Geometry check sheet. Reference: the model listing, model coordinates, mm. A direction names the side the tool comes from. Give positions to 0.01 mm unless a question says otherwise; leave off trailing zeros. Order: outer loops, then holes, each group sorted by start corner. A loop starts at its lowest first (then second) coordinate and runs counter-clockwise, first axis right, second up. Notation, with made-up numbers: M -29,11.5 L 21,11.5 A9 ccw 21,25.5 Z; hole C 49,67 d4. An arc over 180 degrees is marked long. Answer as a JSON object with one key per item and string values. Group by question number.
from build123d import *

# Parameters (mm, degrees)
DODANIE_WYCI_GNI_CIE1_DEPTH = 20
DODANIE_WYCI_GNI_CIE2_DEPTH = 5
OTW_R_GWINTOWANY_M81_D      = 6.8
OTW_R_GWINTOWANY_M81_DEPTH  = 40
OTW_R_GWINTOWANY_M81_TIP    = 2.042926105
SZKIC4_R                    = 19.05
SZKIC4_R_2                  = 3.25
WYTNIJ_WYCI_GNI_CIE2_DEPTH  = 15
SZKIC4_4_R                  = 19.05
SZKIC4_4_R_2                = 3.25
WYTNIJ_WYCI_GNI_CIE3_DEPTH  = 16.6
SZKIC4_5_R                  = 3.25
WYTNIJ_WYCI_GNI_CIE4_DEPTH  = 49.6
WYTNIJ_WYCI_GNI_CIE6_DEPTH  = 10
OTW_R_GWINTOWANY_M61_D      = 5


with BuildPart() as part:
    # Szkic1 → Dodanie-wyci_gni_cie1 (new body)
    with BuildSketch(Plane.XY):
        with BuildLine():
            Line((-50, 0), (0, 0))
            Line((0, 0), (0, 252.5))
            ThreePointArc((0, 252.5), (-17.5, 270), (0, 287.5))
            Line((0, 287.5), (0, 300))
            Line((0, 300), (-21.900286098, 300))
            Line((-21.900286098, 300), (-50, 283.776622614))
            Line((-50, 283.776622614), (-50, 0))
        make_face()
        with BuildLine():
            Line((0, 252.5), (0, 0))
            Line((0, 0), (50, 0))
            Line((50, 0), (50, 283.776622614))
            Line((50, 283.776622614), (21.900286098, 300))
            Line((21.900286098, 300), (0, 300))
            Line((0, 300), (0, 287.5))
            ThreePointArc((0, 287.5), (12.374368671, 282.374368671), (17.5, 270))
            ThreePointArc((17.5, 270), (12.374368671, 257.625631329), (0, 252.5))
        make_face()
    extrude(amount=DODANIE_WYCI_GNI_CIE1_DEPTH)

    # Szkic1_3 → Dodanie-wyci_gni_cie2 (add)
    with BuildSketch(Plane.XY):
        with BuildLine():
            ThreePointArc((0, 287.5), (-17.5, 270), (0, 252.5))
            Line((0, 252.5), (0, 255))
            ThreePointArc((0, 255), (-15, 270), (0, 285))
            Line((0, 285), (0, 287.5))
        make_face()
        with BuildLine():
            Line((0, 255), (0, 252.5))
            ThreePointArc((0, 252.5), (12.374368671, 257.625631329), (17.5, 270))
            ThreePointArc((17.5, 270), (12.374368671, 282.374368671), (0, 287.5))
            Line((0, 287.5), (0, 285))
            ThreePointArc((0, 285), (10.606601718, 280.606601718), (15, 270))
            ThreePointArc((15, 270), (10.606601718, 259.393398282), (0, 255))
        make_face()
    extrude(amount=DODANIE_WYCI_GNI_CIE2_DEPTH)

    # Otw_r gwintowany M81
    with Locations(Plane(origin=(-35, 0, 10), x_dir=(0, 0, -1), z_dir=(0, -1, 0))):
        with Locations((0, 0), (0, 70)):
            Hole(OTW_R_GWINTOWANY_M81_D / 2, depth=OTW_R_GWINTOWANY_M81_DEPTH)
            with Locations((0, 0, -(OTW_R_GWINTOWANY_M81_DEPTH + OTW_R_GWINTOWANY_M81_TIP / 2))):  # 118° drill point
                Cone(0, OTW_R_GWINTOWANY_M81_D / 2, OTW_R_GWINTOWANY_M81_TIP, mode=Mode.SUBTRACT)

    # Szkic4 → Wytnij-wyci_gni_cie2 (cut)
    # profile 1 of 2: a face of its own
    with BuildSketch(Plane(origin=(0, 0, 0), x_dir=(-1, 0, 0), z_dir=(0, 0, -1))):
        with BuildLine():
            Line((-28.2, 53.4), (-28.2, 0))
            Line((-28.2, 0), (28.2, 0))
            Line((28.2, 0), (28.2, 53.4))
            ThreePointArc((28.2, 53.4), (27.321320344, 55.521320344), (25.2, 56.4))
            Line((25.2, 56.4), (-25.2, 56.4))
            ThreePointArc((-25.2, 56.4), (-27.321320344, 55.521320344), (-28.2, 53.4))
        make_face()
        with Locations((0, 28.2)):
            Circle(SZKIC4_R, mode=Mode.SUBTRACT)
    # profile 2 of 2: a face of its own
    with BuildSketch(Plane(origin=(0, 0, 0), x_dir=(-1, 0, 0), z_dir=(0, 0, -1))):
        with Locations((0, 28.2)):
            Circle(SZKIC4_R)
        with Locations((0, 28.2)):
            Circle(SZKIC4_R_2, mode=Mode.SUBTRACT)
    extrude(amount=-WYTNIJ_WYCI_GNI_CIE2_DEPTH, mode=Mode.SUBTRACT)

    # Szkic4_4 → Wytnij-wyci_gni_cie3 (cut)
    with BuildSketch(Plane(origin=(0, 0, 0), x_dir=(-1, 0, 0), z_dir=(0, 0, -1))):
        with Locations((0, 28.2)):
            Circle(SZKIC4_4_R)
        with Locations((0, 28.2)):
            Circle(SZKIC4_4_R_2, mode=Mode.SUBTRACT)
    extrude(amount=-WYTNIJ_WYCI_GNI_CIE3_DEPTH, mode=Mode.SUBTRACT)

    # Szkic4_5 → Wytnij-wyci_gni_cie4 (cut)
    with BuildSketch(Plane(origin=(0, 0, 0), x_dir=(-1, 0, 0), z_dir=(0, 0, -1))):
        with Locations((0, 28.2)):
            Circle(SZKIC4_5_R)
    extrude(amount=-WYTNIJ_WYCI_GNI_CIE4_DEPTH, mode=Mode.SUBTRACT)

    # Szkic6 → Wytnij-wyci_gni_cie6 (cut)
    with BuildSketch(Plane(origin=(0, 0, 0), x_dir=(-1, 0, 0), z_dir=(0, 0, -1))):
        with BuildLine():
            Line((-45, 228.928061115), (-45, 82.471938885))
            ThreePointArc((-45, 82.471938885), (-43.078190139, 80.039718467), (-40.267443069, 81.346910197))
            Line((-40.267443069, 81.346910197), (-5.067175687, 151.199885246))
            ThreePointArc((-5.067175687, 151.199885246), (-3.997403411, 155.7), (-5.067175687, 160.200114754))
            Line((-5.067175687, 160.200114754), (-40.267443069, 230.053089803))
            ThreePointArc((-40.267443069, 230.053089803), (-43.078190139, 231.360281533), (-45, 228.928061115))
        make_face()
        with BuildLine():
            Line((2.232556931, 145.714200914), (38.342819518, 74.055390936))
            ThreePointArc((38.342819518, 74.055390936), (38.218169264, 71.13215965), (35.663751201, 69.70535651))
            Line((35.663751201, 69.70535651), (-35.663751201, 69.70535651))
            ThreePointArc((-35.663751201, 69.70535651), (-38.218169264, 71.13215965), (-38.342819518, 74.055390936))
            Line((-38.342819518, 74.055390936), (-2.232556931, 145.714200914))
            ThreePointArc((-2.232556931, 145.714200914), (0, 147.089172226), (2.232556931, 145.714200914))
        make_face()
        with BuildLine():
            Line((45, 228.928061115), (45, 82.471938885))
            ThreePointArc((45, 82.471938885), (43.078190139, 80.039718467), (40.267443069, 81.346910197))
            Line((40.267443069, 81.346910197), (5.067175687, 151.199885246))
            ThreePointArc((5.067175687, 151.199885246), (3.997403411, 155.7), (5.067175687, 160.200114754))
            Line((5.067175687, 160.200114754), (40.267443069, 230.053089803))
            ThreePointArc((40.267443069, 230.053089803), (43.078190139, 231.360281533), (45, 228.928061115))
        make_face()
        with BuildLine():
            Line((-40.008452698, 240.649965574), (-2.232556931, 165.685799086))
            ThreePointArc((-2.232556931, 165.685799086), (0, 164.310827774), (2.232556931, 165.685799086))
            Line((2.232556931, 165.685799086), (40.008452698, 240.649965574))
            ThreePointArc((40.008452698, 240.649965574), (39.883802443, 243.57319686), (37.329384381, 245))
            Line((37.329384381, 245), (-37.32938438, 245))
            ThreePointArc((-37.32938438, 245), (-39.883802443, 243.57319686), (-40.008452698, 240.649965574))
        make_face()
    extrude(amount=-WYTNIJ_WYCI_GNI_CIE6_DEPTH, mode=Mode.SUBTRACT)

    # Otw_r gwintowany M61 (through all)
    with Locations(Plane(origin=(23.57, 51.77, 15), x_dir=(-1, 0, 0), z_dir=(0, 0, -1))):
        with Locations((0, 0), (47.14, 0), (47.14, -47.14), (0, -47.14)):
            Hole(OTW_R_GWINTOWANY_M61_D / 2)


solid = part.part
1. Cross-section at C-C (y = 237). Record the cut outline in (x, z), and give its area (3 significant figures).
2. Cross-section at A-A (y = 28.2). Record the cut outline in (x, z).
3. Depth check by flat-ended pin: pin 1 (4 mm diameter, centred on x = -18, z = 6.5, fed in from -Y); pin 2 (3 mm diameter, centred on x = -1, y = 49.5, fed in from -Z); pin 3 (1 mm diameter, centred on x = -27.5, y = 123, fed in from -Z). Enter the tip coordinate at first touch or a pass-through.
4. Access from +Z, -Z, +X, -X, +Y, -Y to the whole of each face (thin tool, end or side, straight path). Record for faces 1 (the flat face through (-22.914, 115.784, 4.93)), 2 (the flat face through (0, 56.4, 7)), 3 (the cylindrical face through (37.867, 20.28, 11.828)).
5. Cross-section at D-D (y = 137). Record the cut outline in (x, z).
6. Release check for a two-part mould opening along Y. For faces 4 (the cylindrical face through (-33.979, 20.28, 13.243)), 5 (the flat face through (0, 300, 10)), 6 (the flat face through (-29, 157, 10)) record: released by +Y, released by -Y, zero draft, split by the parting line, or undercut.
7. Thickness scan on line 1 along Y through (x, z) = (0, 19.3); line 2 along X through (y, z) = (12, 10); line 3 along X through (y, z) = (155, 7.25). Record the ranges inside material, lowest first. Write a range as [from, to].
Report:
{
 "1": {"outline": "M -50,0 L -38.17,0 L -38.17,10 L 38.17,10 L 38.17,0 L 50,0 L 50,20 L -50,20 Z", "area": "1,240 mm2"},
 "2": {"outline": "M -50,0 L -28.2,0 L -28.2,15 L -19.05,15 L -19.05,16.6 L -3.25,16.6 L -3.25,20 L -50,20 Z; M 3.25,16.6 L 19.05,16.6 L 19.05,15 L 28.2,15 L 28.2,0 L 50,0 L 50,20 L 3.25,20 Z; hole C -35,10 d6.8; hole C 35,10 d6.8"},
 "3": {"pin 1": "stops at y = 56.4", "pin 2": "stops at z = 15", "pin 3": "stops at z = 10"},
 "4": {"face 1": "-Z", "face 2": "-Z, -Y", "face 3": "-Y"},
 "5": {"outline": "M -50,0 L -45,0 L -45,10 L -12.22,10 L -12.22,0 L -6.62,0 L -6.62,10 L 6.62,10 L 6.62,0 L 12.22,0 L 12.22,10 L 45,10 L 45,0 L 50,0 L 50,20 L -50,20 Z"},
 "6": {"face 4": "zero draft", "face 5": "released by +Y", "face 6": "undercut"},
 "7": {"line 1": "y = [0, 24.95], [31.45, 252.5], [287.5, 300]", "line 2": "x = [-50, -38.4], [-31.6, -28.2], [28.2, 31.6], [38.4, 50]", "line 3": "x = [-50, -45], [-4.02, 4.02], [45, 50]"}
}
